```python
from build123d import *

# Parameters (mm, degrees)
BOSS_EXTRUDE1_DEPTH = 6
BOSS_EXTRUDE2_START = 19
BOSS_EXTRUDE2_DEPTH = 6
BOSS_EXTRUDE3_START = -19
BOSS_EXTRUDE3_DEPTH = 6
BOSS_EXTRUDE4_START = -39
BOSS_EXTRUDE4_DEPTH = 6
SKETCH7_R           = 7.5
CUT_EXTRUDE1_DEPTH  = 25
SKETCH4_R           = 7.5
CUT_EXTRUDE2_DEPTH  = 73.463784058
SKETCH6_R           = 7.5
CUT_EXTRUDE3_DEPTH  = 10
FILLET1_R           = 5
CHAMFER1_SIZE       = 2


with BuildPart() as part:
    # Sketch1 → Boss-Extrude1 (new, symmetric)
    with BuildSketch(Plane(origin=(0, 0, 0), x_dir=(1, 0, 0), z_dir=(0, 1, 0))):
        with BuildLine():
            Line((-45, 25), (20, 25))
            ThreePointArc((20, 25), (45, 0), (20, -25))
            Line((20, -25), (-45, -25))
            Line((-45, -25), (-45, 25))
        make_face()
    extrude(amount=BOSS_EXTRUDE1_DEPTH, both=True)

    # Sketch2 → Boss-Extrude2 (add, symmetric)
    with BuildSketch(Plane.XY.offset(BOSS_EXTRUDE2_START)):
        with BuildLine():
            Line((-45, 6), (-5, 6))
            Line((-5, 6), (-5, 31))
            ThreePointArc((-5, 31), (-25, 51), (-45, 31))
            Line((-45, 31), (-45, 6))
        make_face()
    extrude(amount=BOSS_EXTRUDE2_DEPTH, both=True)

    # Sketch2_2 → Boss-Extrude3 (add, symmetric)
    with BuildSketch(Plane.XY.offset(BOSS_EXTRUDE3_START)):
        with BuildLine():
            Line((-45, 6), (-5, 6))
            Line((-5, 6), (-5, 31))
            ThreePointArc((-5, 31), (-25, 51), (-45, 31))
            Line((-45, 31), (-45, 6))
        make_face()
    extrude(amount=BOSS_EXTRUDE3_DEPTH, both=True)

    # Sketch3 → Boss-Extrude4 (add, symmetric)
    with BuildSketch(Plane(origin=(0, 0, 0), x_dir=(0, 0, -1), z_dir=(1, 0, 0)).offset(BOSS_EXTRUDE4_START)):
        with BuildLine():
            Line((-25, -6), (25, -6))
            Line((25, -6), (25, -24))
            ThreePointArc((25, -24), (0, -49), (-25, -24))
            Line((-25, -24), (-25, -6))
        make_face()
    extrude(amount=BOSS_EXTRUDE4_DEPTH, both=True)

    # Sketch7 → Cut-Extrude1 (cut, symmetric)
    with BuildSketch(Plane.XY):
        with Locations((-25, 31)):
            Circle(SKETCH7_R)
    extrude(amount=CUT_EXTRUDE1_DEPTH, both=True, mode=Mode.SUBTRACT)

    # Sketch4 → Cut-Extrude2 (cut, through all)
    with BuildSketch(Plane(origin=(0, 0, 0), x_dir=(0, 0, -1), z_dir=(1, 0, 0))):
        with Locations((0, -24)):
            Circle(SKETCH4_R)
    extrude(amount=-CUT_EXTRUDE2_DEPTH, mode=Mode.SUBTRACT)

    # Sketch6 → Cut-Extrude3 (cut, symmetric)
    with BuildSketch(Plane(origin=(0, 0, 0), x_dir=(1, 0, 0), z_dir=(0, 1, 0))):
        with Locations(Location((20, 0, 0), (0, 0, 270))):
            Circle(SKETCH6_R)
    extrude(amount=CUT_EXTRUDE3_DEPTH, both=True, mode=Mode.SUBTRACT)

    # Fillet1
    fillet1_edges = [part.edges().sort_by_distance(p)[0] for p in [
        (-25, 6, 13),
        (-5, 6, 19),
        (-5, 6, -19),
        (-25, 6, -13),
        (-33, -6, 0),
    ]]
    fillet(fillet1_edges, radius=FILLET1_R)

    # Chamfer1
    chamfer1_edges = [part.edges().sort_by_distance(p)[0] for p in [
        (45, 6, 0),
        (10, 6, -25),
        (-25, 51, 25),
        (-25, 51, -25),
        (-45, -49, 0),
        (-33, -49, 0),
        (-33, -17.5, -25),
        (-4, -6, -25),
        (45, -6, 0),
        (-33, -17.5, 25),
        (-4, -6, 25),
        (10, 6, 25),
        (-45, 3.5, -25),
        (-5, 21, -25),
        (-45, 3.5, 25),
        (-5, 21, 25),
        (-31.535533906, -7.464466094, 25),
        (-31.535533906, -7.464466094, -25),
        (-3.535533906, 7.464466094, -25),
        (-3.535533906, 7.464466094, 25),
    ]]
    chamfer(chamfer1_edges, length=CHAMFER1_SIZE)


solid = part.part
```
Input: part model. Units: mm. Frame: model coordinates. A direction names the side the tool comes from. Give positions to 0.01 mm unless a question says otherwise; leave off trailing zeros. Order: outer loops, then holes, each group sorted by start corner. A loop starts at its lowest first (then second) coordinate and runs counter-clockwise, first axis right, second up. Notation, with made-up numbers: M -31.75,32.25 L 18.25,32.25 A15 cw 18.25,46.25 Z; hole C -23,15.25 d11. An arc over 180 degrees is marked long. Return JSON: item names as keys, results as strings.
1) Mould query, pull axis Y, two halves, no side actions, for faces 1 (the face through (-5, 21, -18)), 2 (the face through (-26.63, 23.68, 19.08)), 3 (the face through (43.12, -5.875, 0.509)), 4 (the face through (-26.63, 23.68, -18.92)). Classes: released by +Y, released by -Y, zero draft, split by the parting line, or undercut.
Taken from the geometry:
{"face 1": "zero draft", "face 2": "undercut", "face 3": "released by -Y", "face 4": "undercut"}
2) Line query: L1, parallel to Y at x = -25, z = -18.5; L2, parallel to X at y = 2, z = 0; L3, parallel to Y at x = 14, z = -19. Output: solid intervals per line, ascending. Write a range as [from, to].
Taken from the geometry:
{"L1": "y = [-6, 23.5], [38.5, 51]", "L2": "x = [-45, 12.5], [27.5, 45]", "L3": "y = [-6, 6]"}
3) Access query for faces 5 (the face through (-38.916, -16.564, 0.976)), 6 (the face through (-22, 7, 11)). Directions: +Z, -Z, +X, -X, +Y, -Y. A direction counts if a zero-diameter tool reaches every point of the face in a straight line with its end or side. Return the directions, or none.
Taken from the geometry:
{"face 5": "+X, -X", "face 6": "+X, -X, +Y"}
4) Contact query for flat-ended pins moving along their axis: pin 1 (5 mm diameter, centred on y = 19.5, z = -16.5, fed in from +X); pin 2 (10 mm diameter, centred on y = 39.5, z = -16, fed in from +X); pin 3 (14 mm diameter, centred on x = 21.5, z = 3.5, fed in from -Y). Output: stop coordinate, or through.
Taken from the geometry:
{"pin 1": "stops at x = -5", "pin 2": "stops at x = -5.31", "pin 3": "stops at y = -6"}
5) Section query D-D on z = 6. Count the separate pieces of the cut face and the enclosed holes in it, and give its area (3 significant figures).
Taken from the geometry:
{"separate pieces": "3", "enclosed holes": "0", "area": "1,360 mm2"}
6) Section query C-C on x = 9. Output: boundary loops of the cut face in (y, z).
Taken from the geometry:
{"outline": "M -6,-23 L -4,-25 L 4,-25 L 6,-23 L 6,23 L 4,25 L -4,25 L -6,23 Z"}
7) Section query A-A on x = -25. Output: boundary loops of the cut face in (y, z), and give its area (3 significant figures).
Taken from the geometry:
{"outline": "M -6,-23 L -4,-25 L 23.5,-25 L 23.5,-13 L 11,-13 A5 cw 6,-8 L 6,8 A5 cw 11,13 L 23.5,13 L 23.5,25 L -4,25 L -6,23 Z; M 38.5,-25 L 49,-25 L 51,-23 L 51,-13 L 38.5,-13 Z; M 38.5,13 L 51,13 L 51,23 L 49,25 L 38.5,25 Z", "area": "1,320 mm2"}
8) Section query B-B on z = 0. Output: boundary loops of the cut face in (x, y).
Taken from the geometry:
{"outline": "M -45,-47 L -43,-49 L -35,-49 L -33,-47 L -33,-31.5 L -45,-31.5 Z; M -45,-16.5 L -33,-16.5 L -33,-11 A5 cw -28,-6 L 12.5,-6 L 12.5,6 L -45,6 Z; M 27.5,-6 L 43,-6 L 45,-4 L 45,4 L 43,6 L 27.5,6 Z"}
